Part model, mm, in its own coordinate system. Face numbers are marked on the shaded views. A direction names the side the tool comes from. Round coordinates to 2 decimals unless told otherwise and drop trailing zeros. Write each loop counter-clockwise with the first axis right and the second up, starting at its lowest first coordinate (ties: lowest second). Pieces come first, ordered by that corner, then holes. Notation, with made-up numbers: (80.25, 68) -> (98.25, 68) arc R18 ccw to (98.25, 87) -> close; hole circle Ø6 at (-11.75, 11). An arc over 180 degrees is marked (long way). Use CSV: the item, a comma, the result in double quotes. Start each with the question number.
(1) Probe line 1 (X direction, y = 226.5, z = 0); line 2 (Y direction, x = 6, z = 8); line 3 (X direction, y = 13, z = -1.25). List the from-to ranges inside material, lowest first. Write a range as [from, to].
(2) Saw through at B-B (z = 0). Give the cut face in (x, y).
(3) Saw through at A-A (x = 0). Give the cut face in (y, z).
(4) Saw through at C-C (y = 194). Give the cut face in (x, z).
(5) Drop flat-ended pins along their axis: pin 1 (1.5 mm diameter, centred on x = -4.5, y = 93, fed in from +Z); pin 2 (12 mm diameter, centred on y = 226, z = 9, fed in from -X); pin 3 (8 mm diameter, centred on x = 7, y = 82, fed in from -Z). Give the stop position or say it passes through.
(6) Which spindle directions (+Z, -Z, +X, -X, +Y, -Y) get a long thin tool onto all of the face, cutting with end or side? Do the marked faces 1, 2 and 3. Say none if no direction does.
Autodesk Inventor part; units mm, degrees
ref_plane "YZ Plane" through (0, 0, 0) normal (1, 0, 0) x (0, 1, 0)
ref_plane "XZ Plane" through (0, 0, 0) normal (0, 1, 0) x (-1, 0, 0)
ref_plane "XY Plane" through (0, 0, 0) normal (0, 0, 1) x (1, 0, 0)
sketch "Sketch1" plane through (0, 0, 0) normal (0, 1, 0) x (-1, 0, 0)
  circle A0 centre (0, 0) radius 14
  dimension "d0" = 28
extrude "Extrusion1" add sketch "Sketch1" along normal blind 225
sketch "Sketch2" plane through (0, 225, 0) normal (0, 1, 0) x (1, 0, 0)
  circle A0 centre (0, 0) radius 9.5
  dimension "d3" = 19
extrude "Extrusion2" add sketch "Sketch2" along normal blind 22.5
sketch "Sketch3" plane through (0, 247.5, 0) normal (0, 1, 0) x (1, 0, 0)
  circle A0 centre (0, 0) radius 9.5
  circle A1 centre (0, 0) radius 8
  dimension "d6" = 16
extrude "Extrusion3" add sketch "Sketch3" along normal blind 30 contours A1
thread "Thread1"
sketch "Sketch4" plane through (0, 0, 0) normal (0, -1, 0) x (1, 0, 0)
  circle A0 centre (0, 0) radius 9.5
extrude "Extrusion4" add sketch "Sketch4" along normal blind 22.5
sketch "Sketch5" plane through (0, -22.5, 0) normal (0, -1, 0) x (1, 0, 0)
  circle A0 centre (0, 0) radius 8
extrude "Extrusion5" add sketch "Sketch5" along normal blind 30
thread "Thread2"
properties part number "tie rolls"
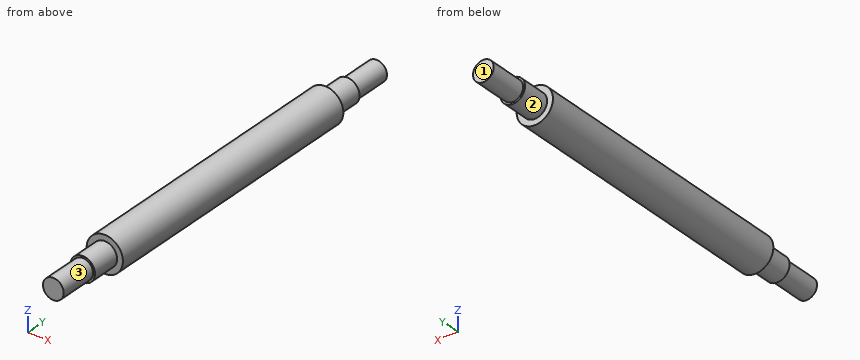
Answers:
1,line 1,"x = [-9.5, 9.5]"
1,line 2,"y = [0, 225]"
1,line 3,"x = [-13.94, 13.94]"
2,outline,"(-14, 0) -> (-9.5, 0) -> (-9.5, -22.5) -> (-8, -22.5) -> (-8, -52.5) -> (8, -52.5) -> (8, -22.5) -> (9.5, -22.5) -> (9.5, 0) -> (14, 0) -> (14, 225) -> (9.5, 225) -> (9.5, 247.5) -> (8, 247.5) -> (8, 277.5) -> (-8, 277.5) -> (-8, 247.5) -> (-9.5, 247.5) -> (-9.5, 225) -> (-14, 225) -> close"
3,outline,"(-52.5, -8) -> (-22.5, -8) -> (-22.5, -9.5) -> (0, -9.5) -> (0, -14) -> (225, -14) -> (225, -9.5) -> (247.5, -9.5) -> (247.5, -8) -> (277.5, -8) -> (277.5, 8) -> (247.5, 8) -> (247.5, 9.5) -> (225, 9.5) -> (225, 14) -> (0, 14) -> (0, 9.5) -> (-22.5, 9.5) -> (-22.5, 8) -> (-52.5, 8) -> close"
4,outline,"circle Ø28 at (0, 0)"
5,pin 1,"stops at z = 13.49"
5,pin 2,"stops at x = -13.66"
5,pin 3,"stops at z = -13.67"
6,face 1,"+Z, -Z, +X, -X, +Y"
6,face 2,"+Y"
6,face 3,"-Y"
